For this review, take the finished solid that the model builds, in its own axes (mm). A direction names the side the tool comes from. Round coordinates to 2 decimals unless told otherwise and drop trailing zeros. Order: outer loops, then holes, each group sorted by start corner. A loop starts at its lowest first (then second) coordinate and runs counter-clockwise, first axis right, second up. Notation, with made-up numbers: (-30, 15) - (20, 15) arc R11 cw to (20, 22) - close; hole circle Ø8 at (63.5, -34). An arc over 180 degrees is marked (long way). Write each question's results on one line, items separated by ' | '. Start each with the question number.
(1) For L1, parallel to X at y = -16, z = -18.5; L2, parallel to X at y = -24.5, z = 1; L3, parallel to X at y = 31.5, z = 1.5, list the stretches that pass through material, from the lowest coordinate up. Write a range as from..to.
(2) Draft analysis for pull direction X (two halves, no side actions). For faces 1 (the cylindrical face through (-19.658, 23.846, 7.509)), 2 (the flat face through (20.273, 1.7, 22.1)), 3 (the cylindrical face through (50.03, 6.14, -11.8)), 4 (the conical face through (7.798, -7.181, 32.337)), state which applies: pulls with the +X half, pulls with the -X half, needs draft (parallel to the pull), parting line crosses it, or undercut.
(3) Take a section at B-B, the plane x = -8.5. Give the boundary of the cut face in (y, z), plus the area to 3 significant figures.
(4) For faces 5 (the flat face through (54.923, 0, 0)), 6 (the cylindrical face through (52.395, 12.932, -5.362)), 7 (the cylindrical face through (21.363, -4.769, -21.477)), list the 3-axis set-ups (+Z, -Z, +X, -X, +Y, -Y) from which the entire face can be reached by the end or side of a thin tool; tool diameter is ignored.
(5) Take a section at A-A, the plane x = 42. Give the boundary of the cut face in (y, z), plus the area to 3 significant figures.
(6) Insertion check: pin 1 Ø2 at (x, z) = (19.5, -7) entering from +Y; pin 2 Ø1.5 at (x, y) = (-11, 21) entering from -Z; pin 3 Ø2 at (x, y) = (7.5, -16) entering from -Z. Each pin has a flat end and moves straight along its axis. Give the tip position at first contact, or say it passes through.
Autodesk Inventor part; units mm, degrees
ref_plane "YZ Plane" through (0, 0, 0) normal (1, 0, 0) x (0, 1, 0)
ref_plane "XZ Plane" through (0, 0, 0) normal (0, 1, 0) x (-1, 0, 0)
ref_plane "XY Plane" through (0, 0, 0) normal (0, 0, 1) x (1, 0, 0)
sketch "pierwsza_proba" plane through (0, 0, 0) normal (0, 0, 1) x (1, 0, 0)
  line L0 (-33.0769, 0) -> (-33.0769, 25)
  line L1 (-26.4269, 23.5) -> (-26.4269, 25)
  line L2 (-13.0769, 25) -> (-13.0769, 35)
  line L3 (-13.0769, 35) -> (7.9231, 35)
  line L4 (7.9231, 35) -> (7.9231, 25)
  line L5 (7.9231, 25) -> (20.2731, 25)
  line L6 (20.2731, 25) -> (20.2731, 22)
  line L7 (20.2731, 22) -> (22.4231, 22)
  line L8 (34.9231, 14) -> (49.2231, 14)
  line L9 (49.2231, 14) -> (49.2231, 13.3)
  line L10 (49.2231, 13.3) -> (50.8231, 13.3)
  line L11 (50.8231, 13.3) -> (50.8231, 14)
  line L12 (50.8231, 14) -> (54.9231, 14)
  line L13 (54.9231, 14) -> (54.9231, 0)
  line L14 (54.9231, 0) -> (-33.0769, 0)
  line L15 (-33.0769, 25) -> (-28.5769, 25)
  line L16 (-28.5769, 25) -> (-28.5769, 23.5)
  line L17 (-28.5769, 23.5) -> (-26.4269, 23.5)
  line L18 (-26.4269, 25) -> (-13.0769, 25)
  line L19 (22.4231, 22) -> (22.4231, 25)
  line L20 (22.4231, 25) -> (26.9231, 25)
  line L21 (34.9231, 14) -> (34.9231, 20)
  line L22 (34.9231, 20) -> (26.9231, 25)
  dimension "d6" = 88
  dimension "d7" = 5.7
  dimension "d12" = 20
  dimension "d13" = 6.65
  dimension "d14" = 70
  dimension "d15" = 50
  dimension "d16" = 47
  dimension "d18" = 28
  dimension "d19" = 26.6
  dimension "d22" = 2.15
  dimension "d23" = 2.15
  dimension "d24" = 44
  dimension "d25" = 28
  dimension "d26" = 28
  dimension "d27" = 1.6
  dimension "d28" = 50
  dimension "d42" = 34.65
  dimension "d43" = 47
  dimension "d44" = 20
  dimension "d45" = 40
revolve "Obrót1" add sketch "pierwsza_proba" angle 360 about axis through (54.9231, 0, 0) along (-1, 0, 0)
chamfer "Faza1" distance 2 angle 45 1 edges at (-33.0769, -25, 0) measured on face at (-33.0769, 2.955, -7.7918)
chamfer "Faza2" distance 2 angle 45 1 edges at (-13.0769, -35, 0) measured on face at (-13.0769, 31.3522, 2.6905)
chamfer "Faza3" distance 2 angle 45 1 edges at (7.9231, -35, 0) measured on face at (7.9231, 31.3522, 2.6905)
chamfer "Faza4" distance 1 angle 45 1 edges at (54.9231, -14, 0) measured on face at (54.9231, -0.0766, 3.7068)
properties part number "Bartosz_Zukowski_model_nr_8.ipj"
Results below:
1) L1: x = -31.62..-28.58, -26.43..20.27, 22.42..27.79 | L2: x = -31.56..-28.58, -26.43..20.27, 22.42..27.69 | L3: x = -13.08..7.92
2) face 1: needs draft | face 2: undercut | face 3: undercut | face 4: pulls with the +X half
3) outline: circle Ø70 at (0, 0) | area: 3,850 mm^2
4) face 5: +Z, -Z, +X, +Y, -Y | face 6: +X | face 7: none
5) outline: circle Ø28 at (0, 0) | area: 616 mm^2
6) pin 1: stops at y = 24.27 | pin 2: stops at z = -28.55 | pin 3: stops at z = -30.59
